from build123d import *

# Parameters (mm, degrees)
SKETCH_1_W          = 24
SKETCH_1_H          = 12
EXTRUDE_1_DEPTH     = 12
SKETCH_2_R          = 1
EXTRUDE_2_DEPTH     = 1.8
SKETCH_3_W          = 24
SKETCH_3_H          = 12
EXTRUDE_3_DEPTH     = 4
EXTRUDE_4_DEPTH     = 4
SKETCH_5_R          = 2
EXTRUDE_5_DEPTH     = 3.5
EXTRUDE_6_DEPTH     = 3
CUT_EXTRUDE_1_DEPTH = 12
SKETCH_9_R          = 3.5
EXTRUDE_7_DEPTH     = 3


with BuildPart() as part:
    # Эскиз1 → Бобышка-Вытянуть1 (new body)
    with BuildSketch(Plane.XY):
        Rectangle(SKETCH_1_W, SKETCH_1_H)
    extrude(amount=EXTRUDE_1_DEPTH)

    # Эскиз2 → Бобышка-Вытянуть2 (add)
    with BuildSketch(Plane(origin=(0, 0, 0), x_dir=(-1, 0, 0), z_dir=(0, 0, -1))):
        with BuildLine():
            Line((12, 6), (15, 6))
            ThreePointArc((15, 6), (15.707106781, 5.707106781), (16, 5))
            Line((16, 5), (16, -5))
            ThreePointArc((16, -5), (15.707106781, -5.707106781), (15, -6))
            Line((15, -6), (12, -6))
            Line((12, -6), (-12, -6))
            Line((-12, -6), (-15, -6))
            ThreePointArc((-15, -6), (-15.707106781, -5.707106781), (-16, -5))
            Line((-16, -5), (-16, 5))
            ThreePointArc((-16, 5), (-15.707106781, 5.707106781), (-15, 6))
            Line((-15, 6), (-12, 6))
            Line((-12, 6), (12, 6))
        make_face()
        with Locations((14, 0)):
            Circle(SKETCH_2_R, mode=Mode.SUBTRACT)
        with Locations((-14, 0)):
            Circle(SKETCH_2_R, mode=Mode.SUBTRACT)
    extrude(amount=EXTRUDE_2_DEPTH)

    # Эскиз3 → Бобышка-Вытянуть3 (add)
    with BuildSketch(Plane(origin=(0, 0, -1.8), x_dir=(-1, 0, 0), z_dir=(0, 0, -1))):
        Rectangle(SKETCH_3_W, SKETCH_3_H)
    extrude(amount=EXTRUDE_3_DEPTH)

    # Эскиз4 → Бобышка-Вытянуть4 (add)
    with BuildSketch(Plane(origin=(0, 0, -5.8), x_dir=(-1, 0, 0), z_dir=(0, 0, -1))):
        with BuildLine():
            ThreePointArc((0.75, 2.90473751), (12, 0), (0.75, -2.90473751))
            ThreePointArc((0.75, -2.90473751), (-3, 0), (0.75, 2.90473751))
        make_face()
    extrude(amount=EXTRUDE_4_DEPTH)

    # Эскиз5 → Бобышка-Вытянуть5 (add)
    with BuildSketch(Plane(origin=(0, 0, -9.8), x_dir=(-1, 0, 0), z_dir=(0, 0, -1))):
        with Locations((6, 0)):
            Circle(SKETCH_5_R)
    extrude(amount=EXTRUDE_5_DEPTH)

    # Эскиз6 → Бобышка-Вытянуть6 (add)
    with BuildSketch(Plane.XY.offset(12)):
        Polygon((12, -6), (12, 6), (-10, 6), (-10, 4), (-12, 4), (-12, -4), (-10, -4), (-10, -6), align=None)
    extrude(amount=EXTRUDE_6_DEPTH)

    # Эскиз8 → Вырез-Вытянуть1 (cut)
    with BuildSketch(Plane(origin=(0, 6, 0), x_dir=(1, 0, 0), z_dir=(0, 1, 0))):
        Polygon((-7, -15), (-12, -12), (-12, -15), align=None)
    extrude(amount=-CUT_EXTRUDE_1_DEPTH, mode=Mode.SUBTRACT)

    # Эскиз9 → Бобышка-Вытянуть7 (add)
    with BuildSketch(Plane.XY.offset(15)):
        with Locations(Location((-6, 0, 0), (0, 0, 253.398450401))):
            Circle(SKETCH_9_R)
    extrude(amount=EXTRUDE_7_DEPTH)


solid = part.part
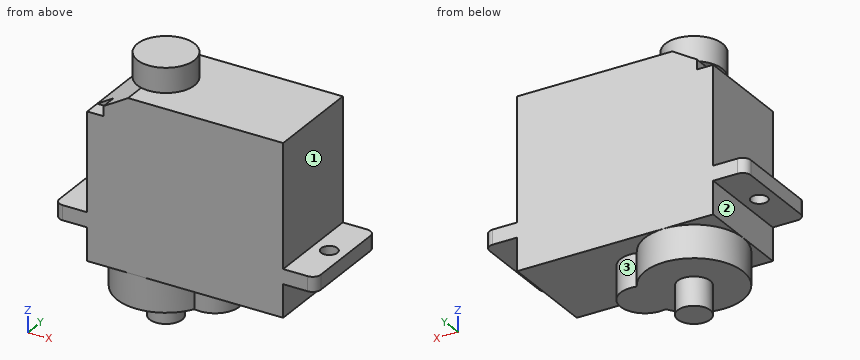
Can you work these out from the model? Positions are in its coordinate system, mm. Face numbers are marked on the shaded views. A direction names the side the tool comes from. Round coordinates to 2 decimals unless told otherwise and drop trailing zeros. Write each loop counter-clockwise with the first axis right and the second up, starting at its lowest first coordinate (ties: lowest second). Pieces come first, ordered by that corner, then holes. Notation, with made-up numbers: M 27.25,27 L 35.25,27 A19 ccw 35.25,46 Z; hole C -4,40 d4. An arc over 180 degrees is marked long. Use a Markdown table: item, result.
Item 1: If I drill on line 1 along Y through (x, z) = (14, -0.95); line 2 along Z through (x, y) = (13, 1.5); line 3 along Z through (x, y) = (-10.5, 4.5), over which ranges is the centre line in solid material (lowest first)? Write a range as [from, to].
Found:
| item | result |
|---|---|
| line 1 | y = [-6, -1], [1, 6] |
| line 2 | z = [-1.8, 0] |
| line 3 | z = [-5.8, 12] |
Item 2: Which directions (+Z, -Z, +X, -X, +Y, -Y) give clear straight access to the entire face, cutting with the end or side of a thin tool? Please do the marked faces 1, 2 and 3.
Found:
| item | result |
|---|---|
| face 1 | +Z, +X, +Y, -Y |
| face 2 | -Z, -X, +Y, -Y |
| face 3 | -Z |
Item 3: I want a section at C-C (y = 0.5). State how many separate pieces and enclosed holes the cut face has, and give its area (3 significant figures).
Found:
| item | result |
|---|---|
| separate pieces | 3 |
| enclosed holes | 0 |
| area | 594 mm2 |
Item 4: I want a section at D-D (z = 3). List the corners of the cut face in (x, y) for me, and give its area (3 significant figures).
Found:
| item | result |
|---|---|
| outline | M -12,-6 L 12,-6 L 12,6 L -12,6 Z |
| area | 288 mm2 |
Item 5: I want a section at B-B (x = 0). List the corners of the cut face in (y, z) for me.
Found:
| item | result |
|---|---|
| outline | M -6,-5.8 L -3,-5.8 L -3,-9.8 L 3,-9.8 L 3,-5.8 L 6,-5.8 L 6,15 L -6,15 Z |
Item 6: I want a section at A-A (x = -14). List the corners of the cut face in (y, z) for me.
Found:
| item | result |
|---|---|
| outline | M -6,-1.8 L -1,-1.8 L -1,0 L -6,0 Z; M 1,-1.8 L 6,-1.8 L 6,0 L 1,0 Z |
Item 7: For pin 1 Ø2 at (y, z) = (1, -4.5) entering from +X; pin 2 Ø3 at (x, y) = (-14, 0) entering from -Z; pin 3 Ø4.5 at (x, y) = (13, -3) entering from -Z, each with a flat end and sliding along its axis, tell me the tip position at first contact or that it passes through.
Found:
| item | result |
|---|---|
| pin 1 | stops at x = 12 |
| pin 2 | stops at z = -1.8 |
| pin 3 | stops at z = -5.8 |
